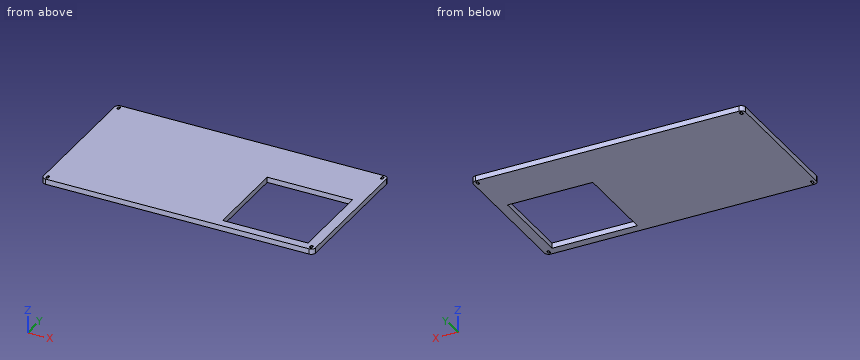
from build123d import *

# Parameters (mm, degrees)
SKETCH1_W           = 647.7
SKETCH1_H           = 343.408
SKETCH1_W_2         = 203.2
SKETCH1_H_2         = 203.2
BOSS_EXTRUDE1_DEPTH = 12.7
FILLET1_R           = 10


with BuildPart() as part:
    # Sketch1 → Boss-Extrude1 (new body)
    with BuildSketch(Plane.XY):
        with Locations((-66.978068182, 49.838840909)):
            Rectangle(SKETCH1_W, SKETCH1_H)
        with BuildLine():
            Line((247.371931818, -116.865159091), (246.371931818, -116.865159091))
            ThreePointArc((246.371931818, -116.865159091), (244.604164865, -116.132926044), (243.871931818, -114.365159091))
            Line((243.871931818, -114.365159091), (243.871931818, -109.365159091))
            ThreePointArc((243.871931818, -109.365159091), (244.604164865, -107.597392138), (246.371931818, -106.865159091))
            Line((246.371931818, -106.865159091), (247.371931818, -106.865159091))
            ThreePointArc((247.371931818, -106.865159091), (249.139698771, -107.597392138), (249.871931818, -109.365159091))
            Line((249.871931818, -109.365159091), (249.871931818, -114.365159091))
            ThreePointArc((249.871931818, -114.365159091), (249.139698771, -116.132926044), (247.371931818, -116.865159091))
        make_face(mode=Mode.SUBTRACT)
        with Locations((131.884838954, 0.072858907)):
            Rectangle(SKETCH1_W_2, SKETCH1_H_2, mode=Mode.SUBTRACT)
        with BuildLine():
            Line((-380.328068182, -116.865159091), (-381.328068182, -116.865159091))
            ThreePointArc((-381.328068182, -116.865159091), (-383.095835135, -116.132926044), (-383.828068182, -114.365159091))
            Line((-383.828068182, -114.365159091), (-383.828068182, -109.365159091))
            ThreePointArc((-383.828068182, -109.365159091), (-383.095835135, -107.597392138), (-381.328068182, -106.865159091))
            Line((-381.328068182, -106.865159091), (-380.328068182, -106.865159091))
            ThreePointArc((-380.328068182, -106.865159091), (-378.560301229, -107.597392138), (-377.828068182, -109.365159091))
            Line((-377.828068182, -109.365159091), (-377.828068182, -114.365159091))
            ThreePointArc((-377.828068182, -114.365159091), (-378.560301229, -116.132926044), (-380.328068182, -116.865159091))
        make_face(mode=Mode.SUBTRACT)
        with BuildLine():
            Line((-380.328068182, 206.544840909), (-381.328068182, 206.544840909))
            ThreePointArc((-381.328068182, 206.544840909), (-383.095835135, 207.277073956), (-383.828068182, 209.044840909))
            Line((-383.828068182, 209.044840909), (-383.828068182, 214.044840909))
            ThreePointArc((-383.828068182, 214.044840909), (-383.095835135, 215.812607862), (-381.328068182, 216.544840909))
            Line((-381.328068182, 216.544840909), (-380.328068182, 216.544840909))
            ThreePointArc((-380.328068182, 216.544840909), (-378.560301229, 215.812607862), (-377.828068182, 214.044840909))
            Line((-377.828068182, 214.044840909), (-377.828068182, 209.044840909))
            ThreePointArc((-377.828068182, 209.044840909), (-378.560301229, 207.277073956), (-380.328068182, 206.544840909))
        make_face(mode=Mode.SUBTRACT)
        with BuildLine():
            Line((247.371931818, 206.544840909), (246.371931818, 206.544840909))
            ThreePointArc((246.371931818, 206.544840909), (244.604164865, 207.277073956), (243.871931818, 209.044840909))
            Line((243.871931818, 209.044840909), (243.871931818, 214.044840909))
            ThreePointArc((243.871931818, 214.044840909), (244.604164865, 215.812607862), (246.371931818, 216.544840909))
            Line((246.371931818, 216.544840909), (247.371931818, 216.544840909))
            ThreePointArc((247.371931818, 216.544840909), (249.139698771, 215.812607862), (249.871931818, 214.044840909))
            Line((249.871931818, 214.044840909), (249.871931818, 209.044840909))
            ThreePointArc((249.871931818, 209.044840909), (249.139698771, 207.277073956), (247.371931818, 206.544840909))
        make_face(mode=Mode.SUBTRACT)
    extrude(amount=BOSS_EXTRUDE1_DEPTH)

    # Fillet1
    fillet1_edges = [part.edges().sort_by_distance(p)[0] for p in [
        (-390.828068182, 221.542840909, 6.35),
        (256.871931818, 221.542840909, 6.35),
        (256.871931818, -121.865159091, 6.35),
        (-390.828068182, -121.865159091, 6.35),
    ]]
    fillet(fillet1_edges, radius=FILLET1_R)


solid = part.part
Design review of the part built by this model. Coordinates are the model's own, in mm. Round coordinates to 2 decimals unless told otherwise and drop trailing zeros. Write each loop counter-clockwise with the first axis right and the second up, starting at its lowest first coordinate (ties: lowest second). Pieces come first, ordered by that corner, then holes.
Item 1: Consider section A-A on y = -26. Give the boundary of the cut face in (x, z), and give its area (3 significant figures).
Item 2: Wall thickness on L1, parallel to Y at x = 116, z = 11.75; L2, parallel to X at y = 31.5, z = 5.5: over which ranges is each line inside the solid? List them lowest first.
Item 3: Consider section C-C on z = 9. Count the separate pieces of the cut face and the enclosed holes in it, and give its area (3 significant figures).
Item 4: For pin 1 Ø2 at (x, y) = (128, 99) entering from -Z, flat-tipped, find the tip position at first contact; note if it passes through.
Item 5: Consider section B-B on x = 208.5. Give the boundary of the cut face in (y, z).
Check values:
1. outline: (-390.83, 0) - (30.28, 0) - (30.28, 12.7) - (-390.83, 12.7) - close; (233.48, 0) - (256.87, 0) - (256.87, 12.7) - (233.48, 12.7) - close
1. area: 5,650 mm2
2. L1: y = -121.87 to -101.53, 101.67 to 221.54
2. L2: x = -390.83 to 30.28, 233.48 to 256.87
3. separate pieces: 1
3. enclosed holes: 5
3. area: 181,000 mm2
4. pin 1: passes through
5. outline: (-121.87, 0) - (-101.53, 0) - (-101.53, 12.7) - (-121.87, 12.7) - close; (101.67, 0) - (221.54, 0) - (221.54, 12.7) - (101.67, 12.7) - close
